from build123d import *

# Parameters (mm, degrees)
PAD_DEPTH    = 25.4
SKETCH001_R  = 2.248154
POCKET_DEPTH = 17.5016


with BuildPart() as part:
    # Sketch → Pad (new body)
    with BuildSketch(Plane.XY):
        with BuildLine():
            ThreePointArc((11.935765, 0.8128), (0, 11.963408), (-11.935765, 0.8128))
            Line((-24.6634, 0.8128), (-11.935765, 0.8128))
            Line((-24.6634, 18.3134), (-24.6634, 0.8128))
            Line((-24.6634, 18.3134), (24.6634, 18.3134))
            Line((24.6634, 18.3134), (24.6634, 0.8128))
            Line((11.935765, 0.8128), (24.6634, 0.8128))
        make_face()
    extrude(amount=PAD_DEPTH)

    # Sketch001 → Pocket (cut, through all)
    with BuildSketch(Plane(origin=(0, 18.3134, 0), x_dir=(-1, 0, 0), z_dir=(0, 1, 0))):
        with Locations((18.3134, 6.35)):
            Circle(SKETCH001_R)
        with Locations((18.3134, 19.05)):
            Circle(SKETCH001_R)
        with Locations((-18.3134, 19.05)):
            Circle(SKETCH001_R)
        with Locations((-18.3134, 6.35)):
            Circle(SKETCH001_R)
    extrude(amount=-POCKET_DEPTH, mode=Mode.SUBTRACT)


solid = part.part
Work out the finished part from the listing and answer in its coordinate system (mm). Give positions to 0.01 mm unless a question says otherwise; leave off trailing zeros. Write each loop counter-clockwise with the first axis right and the second up, starting at its lowest first coordinate (ties: lowest second). Pieces come first, ordered by that corner, then holes. Notation, with made-up numbers: (-33, -33.75) - (-19, -33.75) arc R10 ccw to (-19, -23.75) - close; hole circle Ø6 at (-37.5, 45.25). An arc over 180 degrees is marked (long way). One line per item, written item: value. Start each with the question number.
1. Find section A-A (z = 6.35). Write down the section's boundary in (x, y).
2. Find section B-B (y = 10.75). Write down the section's boundary in (x, z).
3. Find section C-C (x = 19). Write down the section's boundary in (y, z), then the cut area to 3 significant figures.
4. For a pull along X with two mould halves and no side action, classify faces 1 (the flat face through (-18, 0.813, 13)), 2 (the flat face through (24.663, 10, 13)), 3 (the cylindrical face through (0.25, 11.96, 12.52)) as +X half, -X half, draft (parallel to the pull), parting line (faces both ways), or undercut.
5. Consider probe 1 along Z at (x, y) = (20, 14.5); probe 2 along X at (y, z) = (12.25, 19.75); probe 3 along X at (y, z) = (6.75, 13.25). Determine where each line is inside the solid, lowest interval first.
6. Given pin 1 (8 mm diameter, centred on x = -7, y = 14, fed in from -Z), flat-ended and moving along its own axis, determine where the tip first touches the part or whether it passes through.
7. Find section D-D (y = 17.25). Write down the section's boundary in (x, z).
Geometry results:
1. outline: (-24.66, 0.81) - (-20.56, 0.81) - (-20.56, 18.31) - (-24.66, 18.31) - close; (-16.07, 0.81) - (-11.94, 0.81) arc R11.96 cw to (11.94, 0.81) - (16.07, 0.81) - (16.07, 18.31) - (-16.07, 18.31) - close; (20.56, 0.81) - (24.66, 0.81) - (24.66, 18.31) - (20.56, 18.31) - close
2. outline: (-24.66, 0) - (-5.25, 0) - (-5.25, 25.4) - (-24.66, 25.4) - close; (5.25, 0) - (24.66, 0) - (24.66, 25.4) - (5.25, 25.4) - close; hole circle Ø4.5 at (-18.31, 6.35); hole circle Ø4.5 at (-18.31, 19.05); hole circle Ø4.5 at (18.31, 6.35); hole circle Ø4.5 at (18.31, 19.05)
3. outline: (0.81, 0) - (18.31, 0) - (18.31, 4.21) - (0.81, 4.21) - close; (0.81, 8.49) - (18.31, 8.49) - (18.31, 16.91) - (0.81, 16.91) - close; (0.81, 21.19) - (18.31, 21.19) - (18.31, 25.4) - (0.81, 25.4) - close
3. area: 295 mm2
4. face 1: draft
4. face 2: +X half
4. face 3: undercut
5. probe 1: 0 to 4.86, 7.84 to 17.56, 20.54 to 25.4
5. probe 2: -24.66 to -20.45, -16.18 to 16.18, 20.45 to 24.66
5. probe 3: -24.66 to -9.88, 9.88 to 24.66
6. pin 1: z = 0
7. outline: (-24.66, 0) - (24.66, 0) - (24.66, 25.4) - (-24.66, 25.4) - close; hole circle Ø4.5 at (-18.31, 6.35); hole circle Ø4.5 at (-18.31, 19.05); hole circle Ø4.5 at (18.31, 6.35); hole circle Ø4.5 at (18.31, 19.05)
